```python
from build123d import *

# Parameters (mm, degrees)
F1_DEPTH = 50
F3_COUNT = 4
F4_R     = 5


with BuildPart() as f1:
    # F0 (on Right) → F1 (new body, symmetric)
    with BuildSketch(Plane.YZ):
        with BuildLine():
            ThreePointArc((4.996056664, -0.1985391896), (28.756397628, -6.9508107655), (48.0904328859, -22.324231166))
            ThreePointArc((48.0904328859, -22.324231166), (51.6135530474, -22.6202452328), (51.9095671141, -19.0971250713))
            ThreePointArc((51.9095671141, -19.0971250713), (28.6150074029, -1.3179590775), (0, 5))
            ThreePointArc((0, 5), (3.5355339059, 3.5355339059), (5, 0))
            ThreePointArc((5, 0), (4.9990140688, -0.0992891732), (4.996056664, -0.1985391896))
        make_face()
        with BuildLine():
            ThreePointArc((0, 5), (-3.605044795, -3.4646286996), (4.996056664, -0.1985391896))
            ThreePointArc((4.996056664, -0.1985391896), (4.9990140688, -0.0992891732), (5, 0))
            ThreePointArc((5, 0), (3.5355339059, 3.5355339059), (0, 5))
        make_face()
    extrude(amount=F1_DEPTH, both=True)

    # F3: F1 ×4 about axis
    f3_axis = Axis((20.0893953443, 0, 0), (1, 0, 0))


with BuildPart() as f1_1:
    add(f1.part)
    for i in range(1, F3_COUNT):
        add(f1.part.rotate(f3_axis, i * 360 / F3_COUNT))

    # F4
    f4_edges = [f1_1.edges().sort_by_distance(p)[0] for p in [
        (0, 4.999709, -0.19883),
        (0, -0.19883, -4.999709),
        (0, -4.999709, 0.19883),
        (0, 0.19883, 4.999709),
    ]]
    fillet(f4_edges, radius=F4_R)


solid = f1_1.part
```
Geometry: final body of the model. Coordinates: model frame, mm. A direction names the side the tool comes from. Round coordinates to 2 decimals unless told otherwise and drop trailing zeros. Order: outer loops, then holes, each group sorted by start corner. A loop starts at its lowest first (then second) coordinate and runs counter-clockwise, first axis right, second up. Notation, with made-up numbers: (34, 58.5) -> (44, 58.5) arc R27 ccw to (44, 93.5) -> close; hole circle Ø6 at (79.25, 61.5). An arc over 180 degrees is marked (long way). Write each question's results on one line, items separated by ' | '.
Q1. Section query C-C (y = 43). Output: boundary loops of the cut face in (x, z).
Response values:
outline: (-50, -16.97) -> (50, -16.97) -> (50, -10.33) -> (-50, -10.33) -> close
Q2. Pull-direction query (Y, two-part tool) for faces 1 (the face through (0.7, -30.98, 8.15)), 2 (the face through (0.7, -22.655, -51.571)), 3 (the face through (0.7, -51.571, 22.655)), 4 (the face through (-50, 0, 0)); classes: released by +Y, released by -Y, zero draft, split by the parting line, or undercut.
Response values:
face 1: undercut | face 2: split by the parting line | face 3: undercut | face 4: zero draft
Q3. Section query B-B (z = 41). Output: boundary loops of the cut face in (x, y), and give its area (3 significant figures).
Response values:
outline: (-50, 8.76) -> (50, 8.76) -> (50, 15.18) -> (-50, 15.18) -> close | area: 642 mm²
Q4. Access query for faces 5 (the face through (0.7, 31.39, -2.684)), 6 (the face through (0.7, 2.684, 31.39)), 7 (the face through (0.7, -8.15, -30.98)), 8 (the face through (0.7, -2.684, -31.39)). Directions: +Z, -Z, +X, -X, +Y, -Y. A direction counts if a zero-diameter tool reaches every point of the face in a straight line with its end or side. Return the directions, or none.
Response values:
face 5: +X, -X, +Y | face 6: +Z, +X, -X | face 7: +X, -X, -Y | face 8: -Z, +X, -X
Q5. Section query A-A (y = 14). Output: boundary loops of the cut face in (x, z).
Response values:
outline: (-50, -1.58) -> (50, -1.58) -> (50, 3.54) -> (-50, 3.54) -> close; (-50, 39.58) -> (50, 39.58) -> (50, 47.13) -> (-50, 47.13) -> close
Q6. Pin query (flat end, axial travel): pin 1 Ø3 at (x, z) = (-8, 40.5) entering from +Y; pin 2 Ø5 at (x, y) = (-18.5, 33) entering from +Z; pin 3 Ø12 at (x, z) = (28, -27.5) entering from -Y. Return the tip coordinate at first contact, or that it passes through.
Response values:
pin 1: y = 16.06 | pin 2: z = -2.23 | pin 3: y = -9.65
Q7. Ray query, line 1 along Y through (x, z) = (5, -8); line 2 along Z through (x, y) = (-9, -14); line 3 along Y through (x, z) = (43, -10). Return the intervals inside material, ascending.
Response values:
line 1: -1.15 to 4.53, 30.71 to 39.97 | line 2: -47.13 to -39.58, -3.54 to 1.58 | line 3: -0.83 to 4.26, 34.05 to 42.59
